```python
from build123d import *

# Parameters (mm, degrees)
F0_R     = 15.875
F1_DEPTH = 76.2
F2_R     = 15.875
F2_R_2   = 6.35
F3_DEPTH = 44.45
F4_R     = 4.445
F5_DEPTH = 76.2


with BuildPart() as f1:
    # F0 (on Top) → F1 (new body)
    with BuildSketch(Plane.XY):
        Circle(F0_R)
    extrude(amount=F1_DEPTH)

    # F2 (on Top) → F3 (cut)
    with BuildSketch(Plane.XY):
        Circle(F2_R)
        Circle(F2_R_2, mode=Mode.SUBTRACT)
    extrude(amount=F3_DEPTH, mode=Mode.SUBTRACT)

    # F4 (on Right) → F5 (join, symmetric)
    with BuildSketch(Plane.YZ):
        with Locations((0, 60.325)):
            Circle(F4_R)
    extrude(amount=F5_DEPTH, both=True)

    # F7 (on Front) → F8 (revolve)
    with BuildSketch(Plane.XZ):
        with BuildLine():
            Line((76.2, 69.215), (76.2, 51.435))
            ThreePointArc((76.2, 51.435), (85.09, 60.325), (76.2, 69.215))
        make_face()
    revolve(axis=Axis((76.2, 0, 60.325), (0, 0, -1)))

    # F11 (on Front) → F12 (revolve)
    with BuildSketch(Plane.XZ):
        with BuildLine():
            Line((-76.2, 51.435), (-76.2, 69.215))
            ThreePointArc((-76.2, 69.215), (-85.09, 60.325), (-76.2, 51.435))
        make_face()
    revolve(axis=Axis((-76.2, 0, 60.325), (0, 0, -1)))


solid = f1.part
```
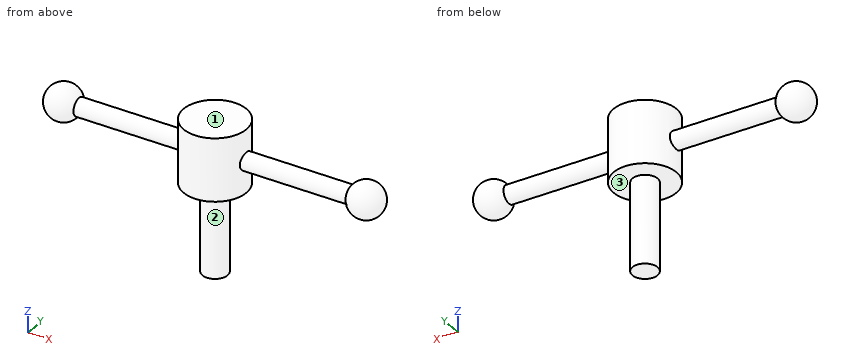
Work out the finished part from the listing and answer in its coordinate system (mm). Face numbers are marked on the shaded views. Round coordinates to 2 decimals unless told otherwise and drop trailing zeros. Loops run counter-clockwise (first coordinate to the right, second up) from the corner with the lowest first, then second, coordinate; pieces in that order, holes last. Notation, with made-up numbers: (-37.75, 41.5) -> (-23.75, 41.5) arc R18 ccw to (-23.75, 56.5) -> close; hole circle Ø7 at (20.5, 17). An arc over 180 degrees is marked (long way). Write each question's results on one line, items separated by ' | '. Start each with the question number.
1. Section D-D (z = 14.5) is taken. Determine the outline of the cut face in (x, y).
2. Section C-C (z = 53) is taken. State how many separate pieces and enclosed holes the cut face has, plus the area to 3 significant figures.
3. Section B-B (y = 0) is taken. Determine the outline of the cut face in (x, z) (3 decimals).
4. For a pull along Z with two mould halves and no side action, classify the marked faces 1, 2 and 3 as +Z half, -Z half, draft (parallel to the pull), parting line (faces both ways), or undercut.
5. Given pin 1 Ø9.5 at (x, y) = (1, 7.5) entering from -Z; pin 2 Ø1.5 at (x, y) = (22, -0.5) entering from +Z; pin 3 Ø2 at (x, y) = (-46, -0.5) entering from -Z; pin 4 Ø1.5 at (y, z) = (-11.5, 49) entering from -X, each flat-ended and moving along its own axis, determine where each tip first touches the part or whether it passes through.
6. Find the intervals of material crossed by probe 1 along X at (y, z) = (-7, 60); probe 2 along X at (y, z) = (-3, 67); probe 3 along Z at (x, y) = (-9, -0.5), in increasing order. Write a range as from..to.
7. Section A-A (x = 0) is taken. Determine the outline of the cut face in (y, z) (3 decimals), plus the area to 3 significant figures.
Evaluation:
1) outline: circle Ø12.7 at (0, 0)
2) separate pieces: 3 | enclosed holes: 0 | area: 951 mm2
3) outline: (-68.501, 55.88) -> (-15.875, 55.88) -> (-15.875, 44.45) -> (-6.35, 44.45) -> (-6.35, 0) -> (6.35, 0) -> (6.35, 44.45) -> (15.875, 44.45) -> (15.875, 55.88) -> (68.501, 55.88) arc R8.89 ccw (long way) to (68.501, 64.77) -> (15.875, 64.77) -> (15.875, 76.2) -> (-15.875, 76.2) -> (-15.875, 64.77) -> (-68.501, 64.77) arc R8.89 ccw (long way) to start
4) face 1: +Z half | face 2: draft | face 3: -Z half
5) pin 1: stops at z = 0 | pin 2: stops at z = 64.77 | pin 3: stops at z = 55.88 | pin 4: stops at x = -11.68
6) probe 1: x = -81.67..-70.73, -14.25..14.25, 70.73..81.67 | probe 2: x = -81.25..-71.15, -15.59..15.59, 71.15..81.25 | probe 3: z = 44.45..76.2
7) outline: (-15.875, 44.45) -> (-6.35, 44.45) -> (-6.35, 0) -> (6.35, 0) -> (6.35, 44.45) -> (15.875, 44.45) -> (15.875, 76.2) -> (-15.875, 76.2) -> close | area: 1,570 mm2
